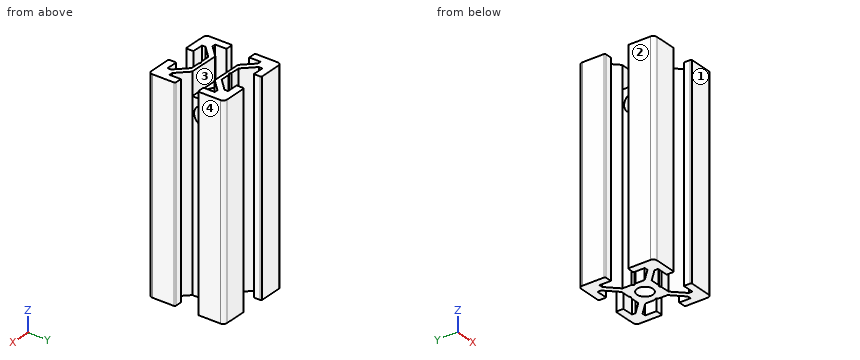
from build123d import *

# Parameters (mm, degrees)
BOSS_EXTRUDE1_DEPTH = 54.5
SKETCH2_W           = 54.5
SKETCH2_H           = 2.1
SKETCH4_R           = 2.5
CUT_EXTRUDE1_DEPTH  = 8
SKETCH5_W           = 6
SKETCH5_H           = 5.999987125
CUT_EXTRUDE2_DEPTH  = 8


with BuildPart() as part:
    # Sketch1 → Boss-Extrude1 (new body)
    with BuildSketch(Plane.XY):
        with BuildLine():
            Line((-10, 9), (-10, 3.29999995))
            ThreePointArc((-10, 3.29999995), (-9.912132049, 3.087867916), (-9.7, 3))
            Line((-9.7, 3), (-8, 3))
            Line((-8, 3), (-8, 6))
            Line((-8, 6), (-7.060677, 6))
            Line((-7.060677, 6), (-4, 2.93932965))
            Line((-4, 2.93932965), (-4, 0.519615242))
            Line((-4, 0.519615242), (-3.699996283, -6.437e-06))
            Line((-3.699996283, -6.437e-06), (-4, -0.519628117))
            Line((-4, -0.519628117), (-4, -2.93933725))
            Line((-4, -2.93933725), (-7.0606695, -6))
            Line((-7.0606695, -6), (-8, -6))
            Line((-8, -6), (-8, -3))
            Line((-8, -3), (-9.7, -3))
            ThreePointArc((-9.7, -3), (-9.912132049, -3.087867916), (-10, -3.29999995))
            Line((-10, -3.29999995), (-10, -9))
            ThreePointArc((-10, -9), (-9.707106781, -9.707106781), (-9, -10))
            Line((-9, -10), (-3.29999995, -10))
            ThreePointArc((-3.29999995, -10), (-3.087867916, -9.912132049), (-3, -9.7))
            Line((-3, -9.7), (-3, -8))
            Line((-3, -8), (-6, -8))
            Line((-6, -8), (-6, -7.0606515))
            Line((-6, -7.0606515), (-2.9393489, -4))
            Line((-2.9393489, -4), (-0.519615242, -4))
            Line((-0.519615242, -4), (6.437e-06, -3.699996283))
            Line((6.437e-06, -3.699996283), (0.519628117, -4))
            Line((0.519628117, -4), (2.9393227, -4))
            Line((2.9393227, -4), (6, -7.060677))
            Line((6, -7.060677), (6, -8))
            Line((6, -8), (3, -8))
            Line((3, -8), (3, -9.7))
            ThreePointArc((3, -9.7), (3.087867916, -9.912132049), (3.29999995, -10))
            Line((3.29999995, -10), (9, -10))
            ThreePointArc((9, -10), (9.707106781, -9.707106781), (10, -9))
            Line((10, -9), (10, -3.29999995))
            ThreePointArc((10, -3.29999995), (9.912132049, -3.087867916), (9.7, -3))
            Line((9.7, -3), (8, -3))
            Line((8, -3), (8, -6))
            Line((8, -6), (7.0606435, -6))
            Line((7.0606435, -6), (4, -2.9393482))
            Line((4, -2.9393482), (4, -0.519615242))
            Line((4, -0.519615242), (3.699996283, 6.437e-06))
            Line((3.699996283, 6.437e-06), (4, 0.519628117))
            Line((4, 0.519628117), (4, 2.9393401))
            Line((4, 2.9393401), (7.060651, 6))
            Line((7.060651, 6), (8, 6))
            Line((8, 6), (8, 3))
            Line((8, 3), (9.7, 3))
            ThreePointArc((9.7, 3), (9.912132049, 3.087867916), (10, 3.29999995))
            Line((10, 3.29999995), (10, 9))
            ThreePointArc((10, 9), (9.707106781, 9.707106781), (9, 10))
            Line((9, 10), (3.29999995, 10))
            ThreePointArc((3.29999995, 10), (3.087867916, 9.912132049), (3, 9.7))
            Line((3, 9.7), (3, 8))
            Line((3, 8), (6, 8))
            Line((6, 8), (6, 7.060669))
            Line((6, 7.060669), (2.9393308, 4))
            Line((2.9393308, 4), (0.519615242, 4))
            Line((0.519615242, 4), (-6.437e-06, 3.699996283))
            Line((-6.437e-06, 3.699996283), (-0.519628117, 4))
            Line((-0.519628117, 4), (-2.93935655, 4))
            Line((-2.93935655, 4), (-6, 7.0606435))
            Line((-6, 7.0606435), (-6, 8))
            Line((-6, 8), (-3, 8))
            Line((-3, 8), (-3, 9.7))
            ThreePointArc((-3, 9.7), (-3.087867966, 9.912132034), (-3.3, 10))
            Line((-3.3, 10), (-9, 10))
            ThreePointArc((-9, 10), (-9.707106781, 9.707106781), (-10, 9))
        make_face()
    extrude(amount=-BOSS_EXTRUDE1_DEPTH)

    # Sketch2 → Cut-Revolve1 (revolve, cut)
    with BuildSketch(Plane(origin=(0, 0, 0), x_dir=(0, 0, -1), z_dir=(1, 0, 0))):
        with Locations((27.25, 1.05)):
            Rectangle(SKETCH2_W, SKETCH2_H)
    revolve(axis=Axis((0, 0, -54.5), (0, 0, 1)), mode=Mode.SUBTRACT)

    # Sketch4 → Cut-Extrude1 (cut)
    with BuildSketch(Plane(origin=(4, 0, 0), x_dir=(0, 0, -1), z_dir=(1, 0, 0))):
        with Locations((10, 6.437e-06)):
            Circle(SKETCH4_R)
    extrude(amount=-CUT_EXTRUDE1_DEPTH, mode=Mode.SUBTRACT)

    # Sketch5 → Cut-Extrude2 (cut)
    with BuildSketch(Plane(origin=(4, 0, 0), x_dir=(0, 0, -1), z_dir=(1, 0, 0))):
        with Locations((3, 6.437e-06)):
            Rectangle(SKETCH5_W, SKETCH5_H)
    extrude(amount=-CUT_EXTRUDE2_DEPTH, mode=Mode.SUBTRACT)


solid = part.part
Source: CAD feature listing. Evaluate the final solid. Frame: model axes, mm. Face numbers are marked on the shaded views. Give positions to 0.01 mm unless a question says otherwise; leave off trailing zeros. Write each loop counter-clockwise with the first axis right and the second up, starting at its lowest first coordinate (ties: lowest second). Pieces come first, ordered by that corner, then holes. Notation, with made-up numbers: M 16,62.25 L 58,62.25 A14 ccw 58,89.25 Z; hole C 82,22 d2. An arc over 180 degrees is marked long. Return JSON: item names as keys, results as strings. Group by question number.
1) Ray query, L1, parallel to X at y = 0, z = -30; L2, parallel to X at y = -9, z = -5. Return the intervals inside material, ascending.
2) First-contact query: pin 1 Ø3 at (y, z) = (-1, -15) entering from +X; pin 2 Ø1.2 at (x, z) = (-2, -35.5) entering from +Y. Flat tips, straight axial feed; report the tip coordinate or a pass-through.
3) Cut plane A-A, the plane y = 1.5. Output: boundary loops of the cut face in (x, z).
4) Draft query along X for the marked faces 1, 2, 3 and 4. Return one class per face: released by +X, released by -X, zero draft, split by the parting line, or undercut.
Data:
{
 "1": {"L1": "x = -3.7 to -2.1, 2.1 to 3.7", "L2": "x = -10 to -3, 3 to 10"},
 "2": {"pin 1": "stops at x = 4", "pin 2": "stops at y = 4"},
 "3": {"outline": "M -4,-54.5 L -1.47,-54.5 L -1.47,-12 L -4,-12 Z; M -4,-8 L -1.47,-8 L -1.47,-6 L -4,-6 Z; M 1.47,-54.5 L 4,-54.5 L 4,-12 L 1.47,-12 Z; M 1.47,-8 L 4,-8 L 4,-6 L 1.47,-6 Z"},
 "4": {"face 1": "zero draft", "face 2": "released by -X", "face 3": "undercut", "face 4": "released by +X"}
}
